Could you check a few things on this model? Use its own coordinates, in mm. Round coordinates to 2 decimals unless told otherwise and drop trailing zeros. Loops run counter-clockwise (first coordinate to the right, second up) from the corner with the lowest first, then second, coordinate; pieces in that order, holes last. Notation, with made-up numbers: (55, 4.25) -> (59, 4.25) arc R18 ccw to (59, 20.25) -> close; hole circle Ø1 at (36.25, 46). An arc over 180 degrees is marked (long way). Write each question's results on one line, items separated by ' | '.
from build123d import *

# Parameters (mm, degrees)
SKETCH2_R           = 2.5
BOSS_EXTRUDE1_DEPTH = 5
FILLET1_R           = 2.5


with BuildPart() as part:
    # Sketch2 → Boss-Extrude1 (new body)
    with BuildSketch(Plane.XY):
        with BuildLine():
            Line((-22.5, 5), (22.5, 5))
            ThreePointArc((22.5, 5), (27.5, 0), (22.5, -5))
            Line((22.5, -5), (-22.5, -5))
            ThreePointArc((-22.5, -5), (-27.5, 0), (-22.5, 5))
        make_face()
        with Locations((-22.5, 0)):
            Circle(SKETCH2_R, mode=Mode.SUBTRACT)
        with Locations(Location((22.5, 0, 0), (0, 0, 180))):
            Circle(SKETCH2_R, mode=Mode.SUBTRACT)
    extrude(amount=BOSS_EXTRUDE1_DEPTH)

    # Fillet1
    fillet1_edges = [part.edges().sort_by_distance(p)[0] for p in [
        (0, -5, 5),
        (0, -5, 0),
        (27.5, 0, 5),
        (27.5, 0, 0),
        (-27.5, 0, 5),
        (-27.5, 0, 0),
        (0, 5, 5),
        (0, 5, 0),
    ]]
    fillet(fillet1_edges, radius=FILLET1_R - 0.0001)  # a hair under: the kernel refuses the full size


solid = part.part
1) I want a section at A-A, the plane y = 0. Give the number of separate pieces and of enclosed holes in the cut face, plus the area to 3 significant figures.
Model answer:
separate pieces: 3 | enclosed holes: 0 | area: 220 mm2
2) I'm going to push a flat-ended pin straight in: pin 1 (4.5 mm diameter, centred on x = 22.5, y = 0, fed in from +Z). Where does the tip first touch, or does it pass through?
Model answer:
pin 1: passes through
3) I want a section at D-D, the plane z = 3.2. Write out the boundary of the cut face in (x, y), plus the area to 3 significant figures.
Model answer:
outline: (-22.5, -4.9) -> (22.5, -4.9) arc R4.9 ccw to (22.5, 4.9) -> (-22.5, 4.9) arc R4.9 ccw to start; hole circle Ø5 at (-22.5, 0); hole circle Ø5 at (22.5, 0) | area: 477 mm2
4) If we mould it in two halves opening along Y, with no side actions, what happens to faces 1 (the flat face through (0, 0, 0)), 2 (the cylindrical face through (0.315, 4.287, 0.752)), 3 (the cylindrical face through (25, 0, 2)), 4 (the cylindrical face through (-25, 0, 2))? For each: released by +Y, released by -Y, zero draft, split by the parting line, or undercut.
Model answer:
face 1: zero draft | face 2: released by +Y | face 3: undercut | face 4: undercut
5) I want a section at B-B, the plane z = 0.9. Write out the boundary of the cut face in (x, y).
Model answer:
outline: (-22.5, -4.42) -> (22.5, -4.42) arc R4.42 ccw to (22.5, 4.42) -> (-22.5, 4.42) arc R4.42 ccw to start; hole circle Ø5 at (-22.5, 0); hole circle Ø5 at (22.5, 0)
6) I need wall thicknesses on line 1 (Y direction, x = 22.5, z = 2.6); line 2 (X direction, y = 2.25, z = 3.95); line 3 (X direction, y = -1.5, z = 2.8). Which ranges of each line are inside material? Lowest first, please.
Model answer:
line 1: y = -5 to -2.5, 2.5 to 5 | line 2: x = -26.44 to -23.59, -21.41 to 21.41, 23.59 to 26.44 | line 3: x = -27.25 to -24.5, -20.5 to 20.5, 24.5 to 27.25
